from build123d import *

# Parameters (mm, degrees)
SKETCH1_R                = 10
BOSS_EXTRUDE1_DEPTH      = 12
BOSS_EXTRUDE2_DEPTH      = 50
BOSS_EXTRUDE3_START      = 12.5
BOSS_EXTRUDE3_DEPTH      = 10
BOSS_EXTRUDE4_DEPTH      = 4
BOSS_EXTRUDE4_DEPTH_BACK = 10
SKETCH3_R                = 15
SKETCH4_R                = 7.5
CUT_EXTRUDE1_DEPTH       = 130.275867818


with BuildPart() as part:
    # Sketch1 → Boss-Extrude1 (new body)
    with BuildSketch(Plane.XY):
        with BuildLine():
            Line((-28.722813233, 20), (-50, 20))
            ThreePointArc((-50, 20), (-68.47759065, 7.653668647), (-64.142135624, -14.142135624))
            Line((-64.142135624, -14.142135624), (-14.142135624, -64.142135624))
            ThreePointArc((-14.142135624, -64.142135624), (0, -70), (14.142135624, -64.142135624))
            Line((14.142135624, -64.142135624), (64.142135624, -14.142135624))
            ThreePointArc((64.142135624, -14.142135624), (68.47759065, 7.653668647), (50, 20))
            Line((50, 20), (28.722813233, 20))
            ThreePointArc((28.722813233, 20), (33.393850206, 10.480971731), (35, 0))
            ThreePointArc((35, 0), (-10.480971731, -33.393850206), (-28.722813233, 20))
        make_face()
        with Locations((0, -50)):
            Circle(SKETCH1_R, mode=Mode.SUBTRACT)
        with Locations((-50, 0)):
            Circle(SKETCH1_R, mode=Mode.SUBTRACT)
        with Locations((50, 0)):
            Circle(SKETCH1_R, mode=Mode.SUBTRACT)
    extrude(amount=BOSS_EXTRUDE1_DEPTH)

    # Sketch1_3 → Boss-Extrude2 (add)
    with BuildSketch(Plane.XY):
        with BuildLine():
            ThreePointArc((28.722813233, 20), (0, 35), (-28.722813233, 20))
            Line((-28.722813233, 20), (-13.971456631, 20))
            ThreePointArc((-13.971456631, 20), (0, 24.39675389), (13.971456631, 20))
            Line((13.971456631, 20), (28.722813233, 20))
        make_face()
        with BuildLine():
            Line((-13.971456631, 20), (-28.722813233, 20))
            ThreePointArc((-28.722813233, 20), (-10.480971731, -33.393850206), (35, 0))
            ThreePointArc((35, 0), (33.393850206, 10.480971731), (28.722813233, 20))
            Line((28.722813233, 20), (13.971456631, 20))
            ThreePointArc((13.971456631, 20), (21.633998582, 11.277043307), (24.39675389, 0))
            ThreePointArc((24.39675389, 0), (-11.277043307, -21.633998582), (-13.971456631, 20))
        make_face()
    extrude(amount=BOSS_EXTRUDE2_DEPTH)

    # Sketch2 → Boss-Extrude3 (add)
    with BuildSketch(Plane(origin=(0, 0, 0), x_dir=(0, 0, -1), z_dir=(1, 0, 0)).offset(BOSS_EXTRUDE3_START)):
        Polygon((-44, 35), (-44, 26.042981562), (-14, 26.042981562), (-14, 55), (-44, 55), align=None)
    extrude(amount=BOSS_EXTRUDE3_DEPTH)

    # Sketch3 → Boss-Extrude4 (add, two sides: drawn at the far end of the back side and taken through both)
    with BuildSketch(Plane(origin=(22.5, 0, 0), x_dir=(0, 0, -1), z_dir=(1, 0, 0)).offset(-BOSS_EXTRUDE4_DEPTH_BACK)):
        with Locations((-29, 55)):
            Circle(SKETCH3_R)
    extrude(amount=BOSS_EXTRUDE4_DEPTH + BOSS_EXTRUDE4_DEPTH_BACK)

    # Sketch4 → Cut-Extrude1 (cut, through all)
    with BuildSketch(Plane(origin=(26.5, 0, 0), x_dir=(0, 0, -1), z_dir=(1, 0, 0))):
        with Locations((-29, 55)):
            Circle(SKETCH4_R)
    extrude(amount=-CUT_EXTRUDE1_DEPTH, mode=Mode.SUBTRACT)

    # Mirror1: part across plane


with BuildPart() as part_1:
    add(part.part)
    add(part.part.mirror(Plane(origin=(0, 0, 0), x_dir=(0, 0, 1), z_dir=(1, 0, 0))))


solid = part_1.part
Input: part model. Units: mm. Frame: model coordinates. A direction names the side the tool comes from. Coordinates: 2 decimals unless noted, no trailing zeros. Loops run counter-clockwise (first coordinate to the right, second up) from the corner with the lowest first, then second, coordinate; pieces in that order, holes last. Notation, with made-up numbers: (-33.75, 55.25) -> (-23.75, 55.25) arc R23 ccw to (-23.75, 79.25) -> close; hole circle Ø11 at (32.25, -12.75). An arc over 180 degrees is marked (long way). Write each question's results on one line, items separated by ' | '. Start each with the question number.
Q1. Section C-C, the plane x = 0. Return the cut outline in (y, z), plus the area to 3 significant figures.
Q2. Section A-A, the plane z = 29. Return the cut outline in (x, y), plus the area to 3 significant figures.
Q3. Pull-direction query (Z, two-part tool) for faces 5 (the cylindrical face through (-19.598, 55.33, 36.493)), 6 (the flat face through (0, -38, 12)), 7 (the flat face through (-26.5, 62, 33)), 8 (the cylindrical face through (20.958, 69.872, 30.953)); classes: released by +Z, released by -Z, zero draft, split by the parting line, or undercut.
Q4. Pin query (flat end, axial travel): pin 1 (5 mm diameter, centred on x = -18.5, y = 36.5, fed in from +Z); pin 2 (8 mm diameter, centred on y = -42.5, z = 22, fed in from +X); pin 3 (15 mm diameter, centred on y = 54, z = 25, fed in from -X); pin 4 (5 mm diameter, centred on x = -15.5, y = 37.5, fed in from -Z). Return the tip coordinate at first contact, or that it passes through.
Q5. Section D-D, the plane x = -16. Return the cut outline in (y, z), plus the area to 3 significant figures.
Q6. Section B-B, the plane y = 57. Return the cut outline in (x, z), plus the area to 3 significant figures.
Q7. Ray query, line 1 (Y direction, x = 0, z = 8); line 2 (Y direction, x = 0, z = 26); line 3 (Y direction, x = 19.5, z = 29). Return the intervals inside material, ascending. Write a range as from..to.
Q8. Reachability of faces 1 (the flat face through (17, 44, 14)), 2 (the flat face through (-12.5, 47, 29)), 3 (the flat face through (-17, 41, 44)), 4 (the flat face through (26.5, 62, 33)) from +Z, -Z, +X, -X, +Y, -Y: full face, straight path, thin tool, end or side. Return the list, or none.
Found:
1) outline: (-70, 0) -> (-60, 0) -> (-60, 12) -> (-70, 12) -> close; (-40, 0) -> (-24.4, 0) -> (-24.4, 50) -> (-35, 50) -> (-35, 12) -> (-40, 12) -> close; (24.4, 0) -> (35, 0) -> (35, 50) -> (24.4, 50) -> close | area: 1,240 mm2
2) outline: (-26.5, 40) -> (-22.5, 40) -> (-22.5, 26.81) arc R35 ccw (long way) to (22.5, 26.81) -> (22.5, 40) -> (26.5, 40) -> (26.5, 47.5) -> (12.5, 47.5) -> (12.5, 32.69) arc R35 ccw to (-12.5, 32.69) -> (-12.5, 47.5) -> (-26.5, 47.5) -> close; (-26.5, 62.5) -> (-12.5, 62.5) -> (-12.5, 70) -> (-26.5, 70) -> close; (12.5, 62.5) -> (26.5, 62.5) -> (26.5, 70) -> (12.5, 70) -> close; hole circle Ø48.79 at (0, 0) | area: 2,600 mm2
3) face 5: undercut | face 6: released by +Z | face 7: zero draft | face 8: split by the parting line
4) pin 1: z = 44 | pin 2: through | pin 3: x = -26.5 | pin 4: z = 14
5) outline: (-62.28, 0) -> (-18.42, 0) -> (-18.42, 50) -> (-31.13, 50) -> (-31.13, 12) -> (-62.28, 12) -> close; (18.42, 0) -> (31.13, 0) -> (31.13, 14) -> (55, 14) arc R15 ccw to (55, 44) -> (31.13, 44) -> (31.13, 50) -> (18.42, 50) -> close; hole circle Ø15 at (55, 29) | area: 2,540 mm2
6) outline: (-26.5, 14.13) -> (-12.5, 14.13) -> (-12.5, 21.77) -> (-26.5, 21.77) -> close; (-26.5, 36.23) -> (-12.5, 36.23) -> (-12.5, 43.87) -> (-26.5, 43.87) -> close; (12.5, 14.13) -> (26.5, 14.13) -> (26.5, 21.77) -> (12.5, 21.77) -> close; (12.5, 36.23) -> (26.5, 36.23) -> (26.5, 43.87) -> (12.5, 43.87) -> close | area: 428 mm2
7) line 1: -70..-60, -40..-24.4, 24.4..35 | line 2: -35..-24.4, 24.4..35 | line 3: -29.06..-14.66, 14.66..47.5, 62.5..70
8) face 1: -Z, +X, +Y | face 2: +Z, -Z, +Y | face 3: +Z, -X, +Y | face 4: +Z, -Z, +X, +Y
